Geometry: see drawing. Coordinates: mm, zero at the bounding-box minimum. Coordinates: 2 decimals unless noted, no trailing zeros. Write each loop counter-clockwise with the first axis right and the second up, starting at its lowest first coordinate (ties: lowest second). Pieces come first, ordered by that corner, then holes.
1) Pin query (flat end, axial travel): pin 1 Ø3 at (x, z) = (36.2, 36.2) entering from -Y. Return the tip coordinate at first contact, or that it passes through.
2) Section query B-B (z = 4.2). Output: boundary loops of the cut face in (x, y).
3) Line query: L1, parallel to Z at x = 4.2, y = 0.4; L2, parallel to X at y = 0.75, z = 36; L3, parallel to Z at x = 37, y = 0.1. Output: solid intervals per line, ascending.
4) Section query A-A (y = 0.15). Output: boundary loops of the cut face in (x, z).
5) Section query C-C (x = 4.2). Output: boundary loops of the cut face in (y, z).
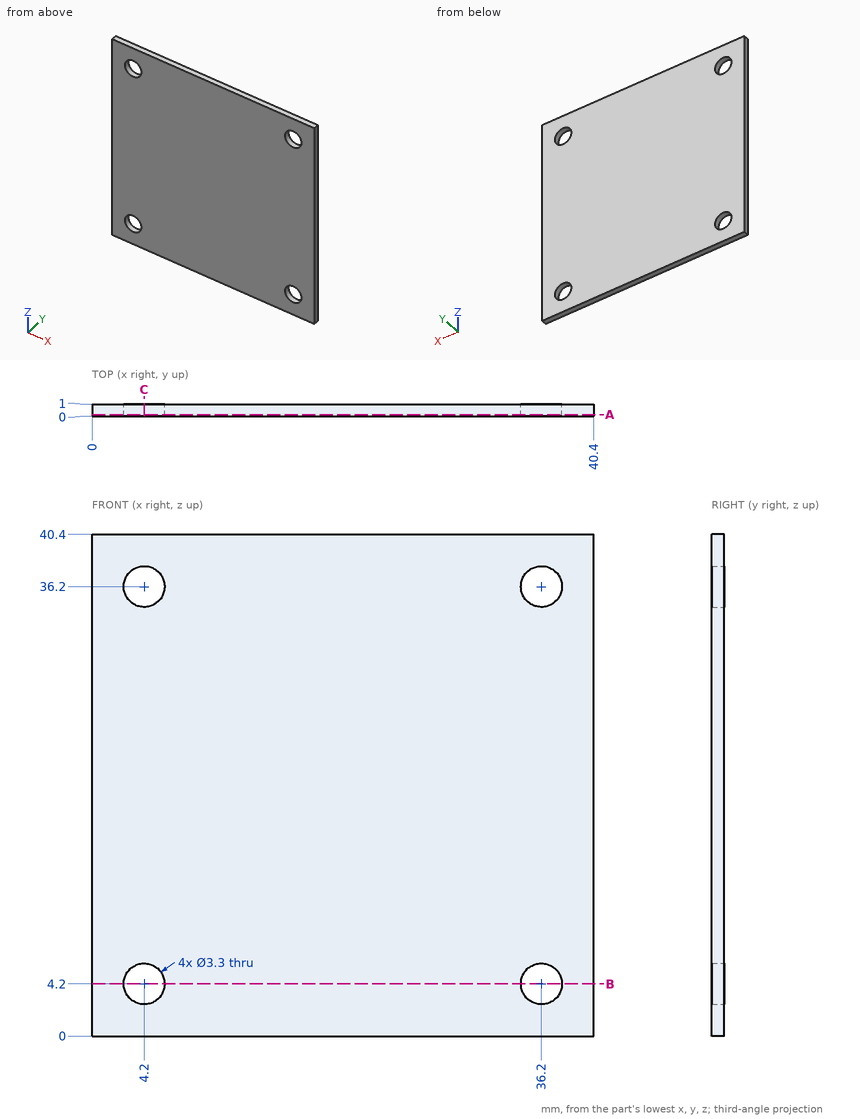
Answer:
1. pin 1: passes through
2. outline: (0, 0) - (2.55, 0) - (2.55, 1) - (0, 1) - close; (5.85, 0) - (34.55, 0) - (34.55, 1) - (5.85, 1) - close; (37.85, 0) - (40.4, 0) - (40.4, 1) - (37.85, 1) - close
3. L1: z = 0 to 2.55, 5.85 to 34.55, 37.85 to 40.4
3. L2: x = 0 to 2.56, 5.84 to 34.56, 37.84 to 40.4
3. L3: z = 0 to 2.76, 5.64 to 34.76, 37.64 to 40.4
4. outline: (0, 0) - (40.4, 0) - (40.4, 40.4) - (0, 40.4) - close; hole circle Ø3.3 at (4.2, 4.2); hole circle Ø3.3 at (4.2, 36.2); hole circle Ø3.3 at (36.2, 4.2); hole circle Ø3.3 at (36.2, 36.2)
5. outline: (0, 0) - (1, 0) - (1, 2.55) - (0, 2.55) - close; (0, 5.85) - (1, 5.85) - (1, 34.55) - (0, 34.55) - close; (0, 37.85) - (1, 37.85) - (1, 40.4) - (0, 40.4) - close
